Geometry: see drawing. Coordinates: mm, zero at the bounding-box minimum. Give positions to 0.01 mm unless a question says otherwise; leave off trailing zeros. Write each loop counter-clockwise with the first axis right and the second up, starting at its lowest first coordinate (ties: lowest second). Pieces come first, ordered by that corner, then holes. Notation, with made-up numbers: M 43.5,80.5 L 75.5,80.5 A31 cw 75.5,113.5 Z; hole C 51,18 d7. An arc over 180 degrees is marked long. Use a Markdown table: item, result. Add a question column.
(1) Draft query along Z for the marked faces 1, 2, 3 and 4. Return one class per face: released by +Z, released by -Z, zero draft, split by the parting line, or undercut.
(2) Pin query (flat end, axial travel): pin 1 Ø5 at (x, z) = (6, 6) entering from +Y. Return the tip coordinate at first contact, or that it passes through.
(3) Cut plane B-B (x = 79). Output: boundary loops of the cut face in (y, z).
(4) Cut plane A-A (z = 6). Output: boundary loops of the cut face in (x, y), plus the area to 3 significant figures.
(5) Cut plane D-D (z = 32). Output: boundary loops of the cut face in (x, y) (1 decimal), plus the area to 4 significant figures.
(6) Material intervals for L1, parallel to X at y = 2.45, z = 6; L2, parallel to X at y = 2.7, z = 24 (1 decimal); L3, parallel to X at y = 1.5, z = 24.5 (1 decimal), sorted ascending.
(7) Cut plane C-C (y = 3). Output: boundary loops of the cut face in (x, z) (1 decimal).
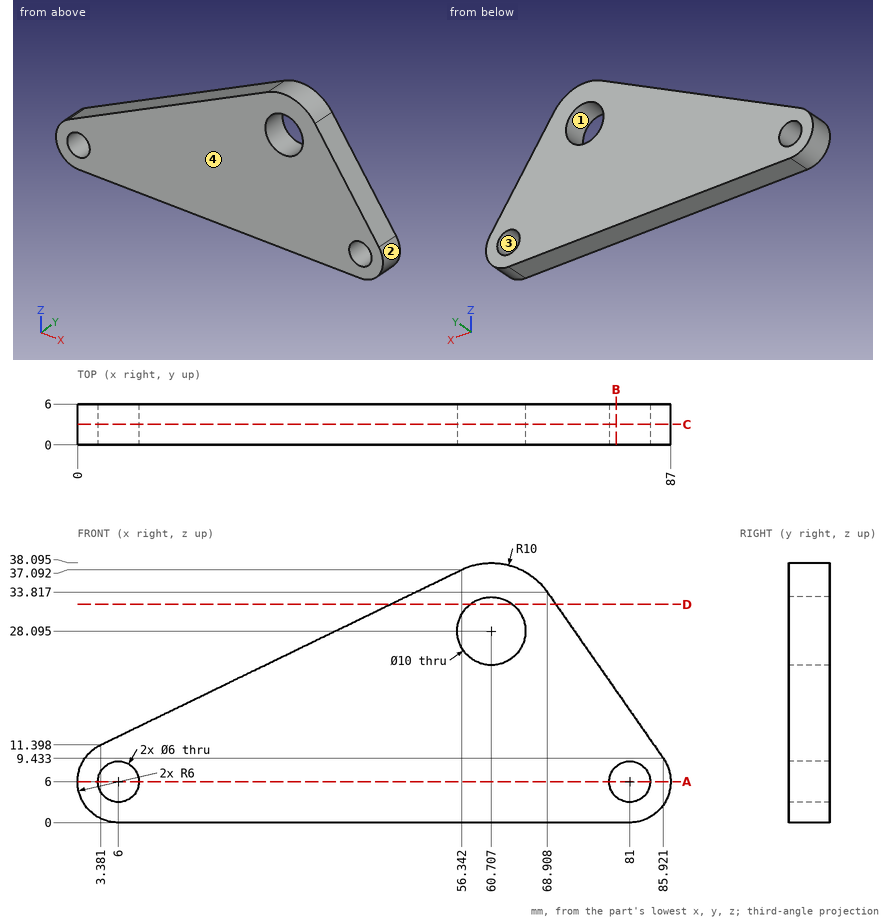
Answer list:
| question | item | result |
|---|---|---|
| 1 | face 1 | undercut |
| 1 | face 2 | split by the parting line |
| 1 | face 3 | undercut |
| 1 | face 4 | zero draft |
| 2 | pin 1 | through |
| 3 | outline | M 0,0 L 6,0 L 6,3.76 L 0,3.76 Z; M 0,8.24 L 6,8.24 L 6,19.35 L 0,19.35 Z |
| 4 | outline | M 0,0 L 3,0 L 3,6 L 0,6 Z; M 9,0 L 78,0 L 78,6 L 9,6 Z; M 84,0 L 87,0 L 87,6 L 84,6 Z |
| 4 | area | 450 mm² |
| 5 | outline | M 45.8,0 L 57.6,0 L 57.6,6 L 45.8,6 Z; M 63.8,0 L 70.2,0 L 70.2,6 L 63.8,6 Z |
| 5 | area | 108.5 mm² |
| 6 | L1 | 0 to 3, 9 to 78, 84 to 87 |
| 6 | L2 | 29.4 to 57.8, 63.6 to 75.8 |
| 6 | L3 | 30.4 to 57.2, 64.2 to 75.4 |
| 7 | outline | M 3.4,11.4 A6 ccw 6,0 L 81,0 A6 ccw 85.9,9.4 L 68.9,33.8 A10 ccw 56.3,37.1 Z; hole C 6,6 d6; hole C 60.7,28.1 d10; hole C 81,6 d6 |
